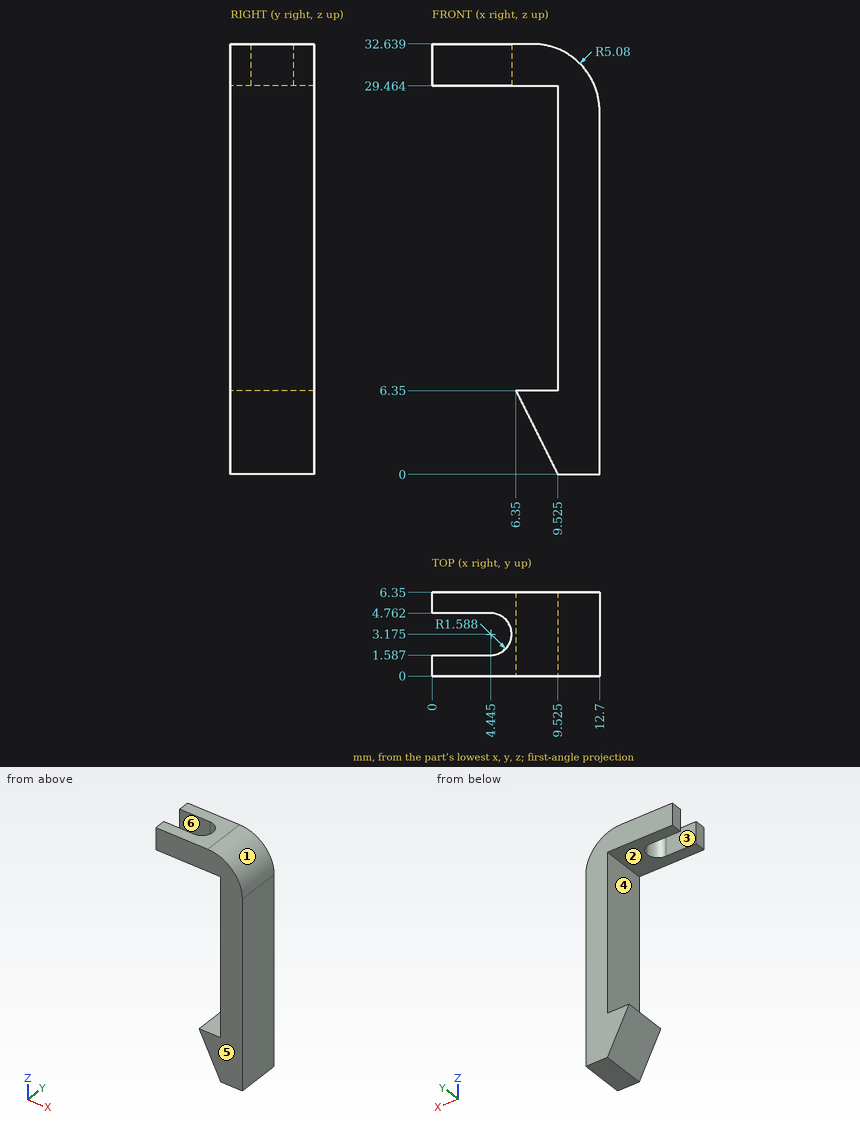
Drawing for the job (mm, zero at the part's lowest x, y, z). A direction names the side the tool comes from. Coordinates: 2 decimals unless noted, no trailing zeros. Use CSV: the item, a comma, the result in double quotes. Start each with the question number.
Q1. 3-axis set-ups, long thin cutter, end or side, ignore diameter. For the marked faces 1, 2 and 3: which of +Z, -Z, +X, -X, +Y, -Y reach the whole face in a straight line?
Q2. Drop flat-ended pins along their axis: P1, Ø1, axis at y = 4, z = 11, coming from the -X side (1 decimal); P2, Ø3, axis at x = 4, y = 3.5, coming from the -Z side. Give the stop position or say it passes through.
Q3. Two-plate mould, pull along Y, no slides. Class the marked faces 4, 5 and 6: +Y half, -Y half, draft (parallel to the pull), parting line (faces both ways), or undercut.
Q4. Probe probe 1 along X at (y, z) = (4.75, 6.5) (1 decimal); probe 2 along Z at (x, y) = (9.75, 3.25); probe 3 along Z at (x, y) = (2, 0.5) (1 decimal). List the from-to ranges inside material, lowest first. Write a range as from..to.
Here are the results:
1,face 1,"+Z, +X, +Y, -Y"
1,face 2,"-X, +Y, -Y"
1,face 3,"+Z, -Z, -X"
2,P1,"x = 9.5"
2,P2,"z = 29.46"
3,face 4,"draft"
3,face 5,"-Y half"
3,face 6,"undercut"
4,probe 1,"9.5..12.7"
4,probe 2,"0..32.17"
4,probe 3,"29.5..32.6"
